Geometry check sheet. Reference: the model listing, model coordinates, mm. A direction names the side the tool comes from. Give positions to 0.01 mm unless a question says otherwise; leave off trailing zeros. Write each loop counter-clockwise with the first axis right and the second up, starting at its lowest first coordinate (ties: lowest second). Pieces come first, ordered by that corner, then holes. Notation, with made-up numbers: (-29.5, 85) -> (7.5, 85) arc R16 cw to (7.5, 111) -> close; hole circle Ø1 at (-11, 86). An arc over 180 degrees is marked (long way). Use a Markdown table: item, result. Add a question column.
from build123d import *

# Parameters (mm, degrees)
SKETCH1_R           = 18.825
BOSS_EXTRUDE1_DEPTH = 57
BOSS_EXTRUDE1_DRAFT = -4.5
SHELL1_T            = -1
SKETCH4_R           = 3.825
CUT_EXTRUDE1_DEPTH  = 57
SKETCH5_W           = 5
SKETCH5_H           = 14
CUT_EXTRUDE2_DEPTH  = 66.846831277
CIRPATTERN1_COUNT   = 12


with BuildPart() as part:
    # Sketch1 → Boss-Extrude1 (with draft: the straight prism first)
    with BuildSketch(Plane(origin=(0, 0, 0), x_dir=(1, 0, 0), z_dir=(0, 1, 0))):
        Circle(SKETCH1_R)
    extrude(amount=BOSS_EXTRUDE1_DEPTH)
    # Boss-Extrude1: the draft: its side faces are tilted about the plane it starts from
    boss_extrude1_sides = [part.faces().sort_by_distance(p)[0] for p in [
        (-18.825, 28.5, 0),
    ]]
    draft(boss_extrude1_sides, Plane(origin=(0, 0, 0), x_dir=(1, 0, 0), z_dir=(0, 1, 0)), BOSS_EXTRUDE1_DRAFT)

    # Shell1
    shell1_openings = [part.faces().sort_by_distance(p)[0] for p in [
        (0, 57, 0),
    ]]
    offset(amount=SHELL1_T, openings=shell1_openings, kind=Kind.INTERSECTION)

    # Sketch4 → Cut-Extrude1 (cut)
    with BuildSketch(Plane.XZ):
        with BuildLine():
            Line((-15.779436777, 1.2), (-12.768736233, 1.2))
            ThreePointArc((-12.768736233, 1.2), (-9.068644469, 9.068644469), (-1.2, 12.768736233))
            Line((-1.2, 12.768736233), (-1.2, 15.779436777))
            ThreePointArc((-1.2, 15.779436777), (-11.189964812, 11.189964812), (-15.779436777, 1.2))
        make_face()
        with BuildLine():
            Line((-1.2, -15.779436777), (-1.2, -12.768736233))
            ThreePointArc((-1.2, -12.768736233), (-9.068644469, -9.068644469), (-12.768736233, -1.2))
            Line((-12.768736233, -1.2), (-15.779436777, -1.2))
            ThreePointArc((-15.779436777, -1.2), (-11.189964812, -11.189964812), (-1.2, -15.779436777))
        make_face()
        with BuildLine():
            Line((15.779436777, -1.2), (12.768736233, -1.2))
            ThreePointArc((12.768736233, -1.2), (9.068644469, -9.068644469), (1.2, -12.768736233))
            Line((1.2, -12.768736233), (1.2, -15.779436777))
            ThreePointArc((1.2, -15.779436777), (11.189964812, -11.189964812), (15.779436777, -1.2))
        make_face()
        with BuildLine():
            ThreePointArc((1.2, 12.768736233), (9.068644469, 9.068644469), (12.768736233, 1.2))
            Line((12.768736233, 1.2), (15.779436777, 1.2))
            ThreePointArc((15.779436777, 1.2), (11.189964812, 11.189964812), (1.2, 15.779436777))
            Line((1.2, 15.779436777), (1.2, 12.768736233))
        make_face()
        with BuildLine():
            Line((-9.751442201, 1.2), (-6.718677325, 1.2))
            ThreePointArc((-6.718677325, 1.2), (-4.826003782, 4.826003782), (-1.2, 6.718677325))
            Line((-1.2, 6.718677325), (-1.2, 9.751442201))
            ThreePointArc((-1.2, 9.751442201), (-6.947324125, 6.947324125), (-9.751442201, 1.2))
        make_face()
        with BuildLine():
            Line((-1.2, -9.751442201), (-1.2, -6.718677325))
            ThreePointArc((-1.2, -6.718677325), (-4.826003782, -4.826003782), (-6.718677325, -1.2))
            Line((-6.718677325, -1.2), (-9.751442201, -1.2))
            ThreePointArc((-9.751442201, -1.2), (-6.947324125, -6.947324125), (-1.2, -9.751442201))
        make_face()
        with BuildLine():
            Line((9.751442201, -1.2), (6.718677325, -1.2))
            ThreePointArc((6.718677325, -1.2), (4.826003782, -4.826003782), (1.2, -6.718677325))
            Line((1.2, -6.718677325), (1.2, -9.751442201))
            ThreePointArc((1.2, -9.751442201), (6.947324125, -6.947324125), (9.751442201, -1.2))
        make_face()
        with BuildLine():
            ThreePointArc((1.2, 6.718677325), (4.826003782, 4.826003782), (6.718677325, 1.2))
            Line((6.718677325, 1.2), (9.751442201, 1.2))
            ThreePointArc((9.751442201, 1.2), (6.947324125, 6.947324125), (1.2, 9.751442201))
            Line((1.2, 9.751442201), (1.2, 6.718677325))
        make_face()
        with Locations(Location((0, 0, 0), (0, 0, 270))):
            Circle(SKETCH4_R)
    extrude(amount=-CUT_EXTRUDE1_DEPTH, mode=Mode.SUBTRACT)

    # Sketch5 → Cut-Extrude2 (cut, through all)
    with BuildSketch(Plane.XY):
        with Locations((0, 8)):
            Rectangle(SKETCH5_W, SKETCH5_H)
        with Locations((0, 28)):
            Rectangle(SKETCH5_W, SKETCH5_H)
    cut_extrude2 = extrude(amount=-CUT_EXTRUDE2_DEPTH, mode=Mode.SUBTRACT)

    # CirPattern1: Cut-Extrude2 ×12 about axis
    cirpattern1_axis = Axis((0, 0, 0), (0, 1, 0))
    for i in range(1, CIRPATTERN1_COUNT):
        add(cut_extrude2.rotate(cirpattern1_axis, i * 360 / CIRPATTERN1_COUNT), mode=Mode.SUBTRACT)


solid = part.part
1) Sectioned sample at A-A, the plane z = 0. Enter the section's corners in (x, y) (3 decimals), and give its area (3 significant figures).
2) Gauge pin test, flat ends, axial feed: P1, Ø6, axis at x = -11, y = 32.5, coming from the +Z side; P2, Ø1.1, axis at x = -18.5, y = 11, coming from the -Z side; P3, Ø0.6, axis at x = 0, z = -21, coming from the -Y side; P4, Ø3.5, axis at x = 9.5, z = 18, coming from the -Y side. Record the tip position at first contact, or that the pin passes through.
3) Material ranges on probe 1 along X at (y, z) = (0.55, 0) (3 decimals); probe 2 along Z at (x, y) = (-18, 39.5); probe 3 along X at (y, z) = (36.5, -10), recorded low to high. Write a range as [from, to].
4) Sectioned sample at B-B, the plane x = 0. Enter the section's corners in (y, z) (3 decimals).
5) Draft check along X on faces 1 (the face through (20.4, 27.9, 2.5)), 2 (the face through (7.221, 7.902, -17.507)), 3 (the face through (-16.381, 27.902, -12.345)), 4 (the face through (-2.5, 27.9, 20.4)). Enter one of: +X half, -X half, draft (parallel to the pull), parting line (faces both ways), or undercut.
6) Tool access check on faces 5 (the face through (7.221, 7.902, 17.507)), 6 (the face through (11.08, 0.49, -11.3)), 7 (the face through (-16.381, 27.902, 12.345)), 8 (the face through (17.507, 7.902, 7.221)). Record the directions out of +Z, -Z, +X, -X, +Y, -Y that give a thin tool (end or side, any length) a straight path to the whole face; none if there is none.
7) Sectioned sample at C-C, the plane y = 40.5. Enter the section's corners in (x, z), and give its area (3 significant figures).
Check values:
| question | item | result |
|---|---|---|
| 1 | outline | (-23.311, 57) -> (-21.58, 35) -> (-20.576, 35) -> (-22.308, 57) -> close; (-20.478, 21) -> (-20.006, 15) -> (-19.002, 15) -> (-19.475, 21) -> close; (-18.904, 1) -> (-18.825, 0) -> (-3.825, 0) -> (-3.825, 1) -> close; (3.825, 0) -> (18.825, 0) -> (18.904, 1) -> (3.825, 1) -> close; (19.002, 15) -> (20.006, 15) -> (20.478, 21) -> (19.475, 21) -> close; (20.576, 35) -> (21.58, 35) -> (23.311, 57) -> (22.308, 57) -> close |
| 1 | area | 86.3 mm² |
| 2 | P1 | z = 19.86 |
| 2 | P2 | z = -7.62 |
| 2 | P3 | y = 35 |
| 2 | P4 | y = 0 |
| 3 | probe 1 | [-18.868, -3.825], [3.825, 18.868] |
| 3 | probe 2 | [-12.53, -10.68], [10.68, 12.53] |
| 3 | probe 3 | [-19.26, -18.12], [18.12, 19.26] |
| 4 | outline | (0, -18.825) -> (1, -18.904) -> (1, -3.825) -> (0, -3.825) -> close; (0, 3.825) -> (1, 3.825) -> (1, 18.904) -> (0, 18.825) -> close; (15, -20.006) -> (21, -20.478) -> (21, -19.475) -> (15, -19.002) -> close; (15, 19.002) -> (21, 19.475) -> (21, 20.478) -> (15, 20.006) -> close; (35, -21.58) -> (57, -23.311) -> (57, -22.308) -> (35, -20.576) -> close; (35, 20.576) -> (57, 22.308) -> (57, 23.311) -> (35, 21.58) -> close |
| 5 | face 1 | draft |
| 5 | face 2 | +X half |
| 5 | face 3 | -X half |
| 5 | face 4 | undercut |
| 6 | face 5 | +X |
| 6 | face 6 | +Y, -Y |
| 6 | face 7 | -X |
| 6 | face 8 | +Z |
| 7 | outline | circle Ø44.02 at (0, 0); hole circle Ø42.02 at (0, 0) |
| 7 | area | 136 mm² |
